Build history of the part. All positions in model axes, mm. A direction names the side the tool comes from. Give positions to 0.01 mm unless a question says otherwise; leave off trailing zeros. Order: outer loops, then holes, each group sorted by start corner. A loop starts at its lowest first (then second) coordinate and runs counter-clockwise, first axis right, second up. Notation, with made-up numbers: (12, 27.25) - (39, 27.25) arc R7 cw to (39, 36.25) - close; hole circle Ø4 at (85, 31). An arc over 180 degrees is marked (long way). Use a Markdown table: item, result.
from build123d import *

# Parameters (mm, degrees)
CROQUIS3_R                   = 20
SALIENTE_EXTRUIR1_DEPTH      = 30
CROQUIS4_W                   = 100
CROQUIS4_H                   = 50
SALIENTE_EXTRUIR2_DEPTH      = 65
CROQUIS5_W                   = 100
CROQUIS5_H                   = 50
SALIENTE_EXTRUIR3_DEPTH      = 35
SALIENTE_EXTRUIR4_DEPTH      = 15
SALIENTE_EXTRUIR4_DEPTH_BACK = 15
REDONDEO2_R                  = 50


with BuildPart() as part:
    # Croquis3 → Saliente-Extruir1 (new body)
    with BuildSketch(Plane(origin=(0, 0, 0), x_dir=(1, 0, 0), z_dir=(0, 1, 0))):
        with BuildLine():
            Line((-50, 0), (-50, -50))
            Line((-50, -50), (50, -50))
            Line((50, -50), (50, 0))
            ThreePointArc((50, 0), (0, 50), (-50, 0))
        make_face()
        with Locations(Location((0, 0, 0), (0, 0, 270))):
            Circle(CROQUIS3_R, mode=Mode.SUBTRACT)
    extrude(amount=SALIENTE_EXTRUIR1_DEPTH)

    # Croquis4 → Saliente-Extruir2 (add)
    with BuildSketch(Plane(origin=(0, 0, 0), x_dir=(1, 0, 0), z_dir=(0, 1, 0))):
        with Locations((0, -75)):
            Rectangle(CROQUIS4_W, CROQUIS4_H)
    extrude(amount=SALIENTE_EXTRUIR2_DEPTH)

    # Croquis5 → Saliente-Extruir3 (add)
    with BuildSketch(Plane.XZ):
        with Locations((0, 75)):
            Rectangle(CROQUIS5_W, CROQUIS5_H)
    extrude(amount=SALIENTE_EXTRUIR3_DEPTH)

    # Croquis6 → Saliente-Extruir4 (add, two sides: drawn at the far end of the back side and taken through both)
    with BuildSketch(Plane(origin=(0, 0, 0), x_dir=(0, 0, -1), z_dir=(1, 0, 0)).offset(-SALIENTE_EXTRUIR4_DEPTH_BACK)):
        with BuildLine():
            Line((-100, 65), (-193.3, 65))
            Line((-193.3, 65), (-193.3, 40))
            Line((-193.3, 40), (-150, 40))
            ThreePointArc((-150, 40), (-125, 15), (-150, -10))
            Line((-150, -10), (-193.3, -10))
            Line((-193.3, -10), (-193.3, -35))
            Line((-193.3, -35), (-100, -35))
            Line((-100, -35), (-100, 65))
        make_face()
    extrude(amount=SALIENTE_EXTRUIR4_DEPTH + SALIENTE_EXTRUIR4_DEPTH_BACK)

    # Redondeo2
    # the kernel refuses this fillet: 50 mm, written as the material it takes off along each edge
    with BuildSketch(Plane(origin=(123.253175473, -35, 193.3), x_dir=(0, 0, -1), z_dir=(-1, 0, 0)), Plane(origin=(-123.253175473, 65, 193.3), x_dir=(0, 0, -1), z_dir=(1, 0, 0))) as redondeo2_piece_1:
        with BuildLine():
            CenterArc((43.301270189, -50), REDONDEO2_R, 90, 60)
            Line((0, -25), (-0.866025404, -24.5))
            ThreePointArc((-0.866025404, -24.5), (-1, -12.5), (-1, 0))
            Line((-1, 0), (0, 1))
            Line((0, 1), (43.301270189, 1))
            Line((43.301270189, 1), (43.301270189, 0))
        make_face()
    extrude(amount=246.506350946, mode=Mode.SUBTRACT)


solid = part.part
1) Wall check: line 1 (X direction, y = 15, z = 0); line 2 (X direction, y = -15.5, z = 121.5); line 3 (Z direction, x = 28, y = 46). Give the ranges that are in metal, low to high. Write a range as from..to.
Computed:
| item | result |
|---|---|
| line 1 | x = -50..-20, 20..50 |
| line 2 | x = -15..15 |
| line 3 | z = 50..100 |
2) Slice it at A-A (y = 15). Write the cut outline in (x, z), and give its area (3 significant figures).
Computed:
| item | result |
|---|---|
| outline | (-50, 0) arc R50 ccw to (50, 0) - (50, 100) - (15, 100) - (15, 125) - (-15, 125) - (-15, 100) - (-50, 100) - close; hole circle Ø40 at (0, 0) |
| area | 13,400 mm² |
3) Two-plate mould, pull along Y, no slides. Class faces 6 (the flat face through (-1, 30, 22)), 7 (the flat face through (32, 16, 100)), 8 (the cylindrical face through (-0.21, 15.55, 125.006)), 9 (the flat face through (0, -10, 171)): +Y half, -Y half, draft (parallel to the pull), parting line (faces both ways), or undercut.
Computed:
| item | result |
|---|---|
| face 6 | +Y half |
| face 7 | draft |
| face 8 | undercut |
| face 9 | undercut |
4) Slice it at C-C (z = 153). Write the cut outline in (x, y).
Computed:
| item | result |
|---|---|
| outline | (-15, -34.91) - (15, -34.91) - (15, -10) - (-15, -10) - close; (-15, 40) - (15, 40) - (15, 64.91) - (-15, 64.91) - close |
5) Slice it at B-B (x = 0). Write the cut outline in (y, z), and give its area (3 significant figures).
Computed:
| item | result |
|---|---|
| outline | (-35, 50) - (0, 50) - (0, 20) - (30, 20) - (30, 50) - (65, 50) - (65, 150) arc R50 ccw to (40, 193.3) - (40, 150) arc R25 cw to (-10, 150) - (-10, 193.3) arc R50 ccw to (-35, 150) - close; (0, -50) - (30, -50) - (30, -20) - (0, -20) - close |
| area | 12,400 mm² |
6) Tool access for faces 1 (the flat face through (-1, 47, 50)), 2 (the flat face through (-1, 0, 22)), 3 (the flat face through (-1, 65, 88)), 4 (the flat face through (-33, 16, 100)), 5 (the flat face through (15, 27, 127)): list every direction of +Z, -Z, +X, -X, +Y, -Y with a clear straight run to the whole face (end or side of a thin tool).
Computed:
| item | result |
|---|---|
| face 1 | -Z, +X, -X, +Y |
| face 2 | -Z, +X, -X, -Y |
| face 3 | +Z, -Z, +X, -X, +Y |
| face 4 | +Z, -X, +Y, -Y |
| face 5 | +Z, +X, +Y, -Y |
7) Slice it at D-D (x = 32). Write the cut outline in (y, z).
Computed:
| item | result |
|---|---|
| outline | (-35, 50) - (0, 50) - (0, -38.42) - (30, -38.42) - (30, 50) - (65, 50) - (65, 100) - (-35, 100) - close |
8) Pin check, flat tips, straight feed: P1, Ø24, axis at x = -6.5, z = 163.5, coming from the +Y side; P2, Ø24, axis at x = -5, z = 181.5, coming from the -Y side; P3, Ø1.5, axis at x = -11.5, z = 153, coming from the -Y side. Stop position of each tip, or through.
Computed:
| item | result |
|---|---|
| P1 | stops at y = 64.98 |
| P2 | stops at y = -31.04 |
| P3 | stops at y = -34.95 |
